from build123d import *
from build123d.topology import SkipClean

# Parameters (mm, degrees)
CUT_EXTRUDE3_DEPTH = 44.910420176
CUT_EXTRUDE7_DEPTH = 44.910420261
FILLET1_R          = 1


with BuildPart() as part:
    # Sketch1 → Revolve1 (revolve)
    with BuildSketch(Plane.XY, mode=Mode.PRIVATE) as revolve1_sk:
        with BuildLine():
            Line((-18.75, 0), (-18.75, 17.954213104))
            ThreePointArc((-18.75, 17.954213104), (-10.400153842, 18.968523534), (-2, 19.4))
            Line((-2, 19.4), (-2, 35))
            Line((-2, 35), (0, 35))
            Line((0, 35), (0, 17.416538555))
            ThreePointArc((0, 17.416538555), (-8.395945025, 17.119829186), (-16.75, 16.231181456))
            Line((-16.75, 16.231181456), (-16.75, 0))
            Line((-16.75, 0), (-18.75, 0))
        make_face()
    revolve(revolve1_sk.sketch.rotate(Axis((0, -0.123973159, 0), (0, 1, 0)), 270), axis=Axis((0, -0.123973159, 0), (0, 1, 0)))

    # Sketch2 → Cut-Extrude3 (cut, through all)
    with SkipClean():  # the faces are left unmerged after this step: merging them gives an invalid solid
        with BuildSketch(Plane(origin=(0, 35, 0), x_dir=(1, 0, 0), z_dir=(0, 1, 0))):
            with BuildLine():
                Line((-13.950632511, 9.270509831), (-6.735419649, 9.270509831))
                Line((-6.735419649, 9.270509831), (-4.505796256, 16.132585041))
                ThreePointArc((-4.505796256, 16.132585041), (-9.845402976, 13.551034656), (-13.950632511, 9.270509831))
            make_face()
            with BuildLine():
                ThreePointArc((-16.735367744, 0.69997605), (-15.930196648, -5.176034656), (-13.127761313, -10.403094872))
                Line((-13.127761313, -10.403094872), (-10.89813792, -3.541019662))
                Line((-10.89813792, -3.541019662), (-16.735367744, 0.69997605))
            make_face()
            with BuildLine():
                Line((0, -11.458980338), (-5.837229824, -15.69997605))
                ThreePointArc((-5.837229824, -15.69997605), (0, -16.75), (5.837229824, -15.69997605))
                Line((5.837229824, -15.69997605), (0, -11.458980338))
            make_face()
            with BuildLine():
                Line((16.735367744, 0.69997605), (10.89813792, -3.541019662))
                Line((10.89813792, -3.541019662), (13.127761313, -10.403094872))
                ThreePointArc((13.127761313, -10.403094872), (15.818541367, -5.507835238), (16.75, 0))
                ThreePointArc((16.75, 0), (16.746341536, 0.350064485), (16.735367744, 0.69997605))
            make_face()
            with BuildLine():
                Line((4.505796256, 16.132585041), (6.735419649, 9.270509831))
                Line((6.735419649, 9.270509831), (13.950632511, 9.270509831))
                ThreePointArc((13.950632511, 9.270509831), (9.845402976, 13.551034656), (4.505796256, 16.132585041))
            make_face()
        extrude(amount=-CUT_EXTRUDE3_DEPTH, mode=Mode.SUBTRACT)
    add(part.part.scale(1), mode=Mode.REPLACE)  # the faces are merged on a copy

    # Sketch3 → Cut-Extrude7 (cut, through all)
    with BuildSketch(Plane(origin=(0, 35, 0), x_dir=(1, 0, 0), z_dir=(0, 1, 0))):
        with BuildLine():
            ThreePointArc((-14.098050985, 4.080734444), (-14.279686617, 4.639751438), (-13.804158359, 4.985242941))
            Line((-13.804158359, 4.985242941), (-4.828377885, 4.985242941))
            Line((-4.828377885, 4.985242941), (-6.836492044, -1.195096947))
            Line((-6.836492044, -1.195096947), (-14.098050985, 4.080734444))
        make_face()
        with BuildLine():
            ThreePointArc((-0.475528258, 14.653742885), (0, 14.999234388), (0.475528258, 14.653742885))
            Line((0.475528258, 14.653742885), (3.249196962, 6.117268377))
            Line((3.249196962, 6.117268377), (-3.249196962, 6.117268377))
            Line((-3.249196962, 6.117268377), (-0.475528258, 14.653742885))
        make_face()
        with BuildLine():
            Line((6.821925031, -1.199830056), (14.083483972, 4.076001334))
            ThreePointArc((14.083483972, 4.076001334), (14.265119604, 4.635018328), (13.789591346, 4.980509831))
            Line((13.789591346, 4.980509831), (4.813810872, 4.980509831))
            Line((4.813810872, 4.980509831), (6.821925031, -1.199830056))
        make_face()
        with BuildLine():
            ThreePointArc((8.997964401, -11.575618528), (8.816328769, -12.134635522), (8.228543517, -12.134635522))
            Line((8.228543517, -12.134635522), (0.966984575, -6.858804132))
            Line((0.966984575, -6.858804132), (6.224295697, -3.03914402))
            Line((6.224295697, -3.03914402), (8.997964401, -11.575618528))
        make_face()
        with BuildLine():
            ThreePointArc((-8.228543517, -12.134635522), (-8.816328769, -12.134635522), (-8.997964401, -11.575618528))
            Line((-8.997964401, -11.575618528), (-6.224295697, -3.03914402))
            Line((-6.224295697, -3.03914402), (-0.966984575, -6.858804132))
            Line((-0.966984575, -6.858804132), (-8.228543517, -12.134635522))
        make_face()
    extrude(amount=-CUT_EXTRUDE7_DEPTH, mode=Mode.SUBTRACT)

    # Fillet1
    fillet1_edges = [part.edges().sort_by_distance(p)[0] for p in [
        (0, 17.954213104, 18.75),
    ]]
    fillet(fillet1_edges, radius=FILLET1_R)


solid = part.part
CAD build for the part. Positions are in the model's coordinates, mm. Round coordinates to 2 decimals unless told otherwise and drop trailing zeros. Order: outer loops, then holes, each group sorted by start corner. A loop starts at its lowest first (then second) coordinate and runs counter-clockwise, first axis right, second up. Notation, with made-up numbers: (15.5, 50.5) -> (45.5, 50.5) arc R17 cw to (45.5, 78.5) -> close; hole circle Ø10 at (32, -29.75). An arc over 180 degrees is marked (long way). Write each question's results on one line, items separated by ' | '.
1. Cut at A-A (z = 9). Count the separate pieces of the cut face and the enclosed holes in it, plus the area to 3 significant figures.
Findings below:
separate pieces: 5 | enclosed holes: 0 | area: 118 mm²
2. Pull direction X, two halves, no side cores. Call faces 1 (the face through (-15.4, 0, -7)), 2 (the face through (11.41, 8.67, 14.88)), 3 (the face through (-13.776, 17.57, 1.45)), 4 (the face through (11.997, 17.57, 6.924)): pulls with the +X half, pulls with the -X half, needs draft (parallel to the pull), parting line crosses it, or undercut.
Findings below:
face 1: needs draft | face 2: parting line crosses it | face 3: undercut | face 4: undercut
3. Flat gauge pins, fed straight in: P1, Ø6, axis at y = 16.5, z = 1.5, coming from the +X side; P2, Ø12, axis at x = -7.5, z = -5.5, coming from the +Y side; P3, Ø5, axis at x = 10, y = 20, coming from the +Z side; P4, Ø2.5, axis at x = 1, y = 18.5, coming from the -Z side. Where does each tip first touch, or does it go through?
Findings below:
P1: stops at x = 18.75 | P2: stops at y = 19.37 | P3: stops at z = 16.22 | P4: stops at z = -18.72
4. Cut at C-C (y = 24.5). Give the cut face in (x, z).
Findings below:
outline: circle Ø4 at (0, 0)
5. Wall check: line 1 along Z through (x, y) = (-0.5, 11); line 2 along X through (y, z) = (17.5, -3.5); line 3 along X through (y, z) = (17.5, 10.5). Give the ranges that are in metal, low to high. Write a range as [from, to].
Findings below:
line 1: z = [-18.74, -16.74], [16.74, 18.74] | line 2: x = [-18.33, -13.3], [-5.31, 5.29], [13.29, 18.33] | line 3: x = [-15.43, -8.65], [-5.98, 5.98], [8.65, 15.43]
